Build history of the part. All positions in model axes, mm. Face numbers are marked on the shaded views. A direction names the side the tool comes from. Coordinates: 2 decimals unless noted, no trailing zeros. Loops run counter-clockwise (first coordinate to the right, second up) from the corner with the lowest first, then second, coordinate; pieces in that order, holes last.
Item 1: 3-axis set-ups, long thin cutter, end or side, ignore diameter. For the marked faces 1, 2 and 3: which of +Z, -Z, +X, -X, +Y, -Y reach the whole face in a straight line?
Item 2: Cut at A-A (y = 0.5). List the corners of the cut face in (x, z).
Item 3: Mould opens along X. For the marked faces 4, 5, 6 and 7 say: released by +X, released by -X, zero draft, split by the parting line, or undercut.
Item 4: Flat gauge pins, fed straight in: pin 1 (1.8 mm diameter, centred on x = -14, y = -28.5, fed in from -Z); pin 2 (3 mm diameter, centred on x = 14, y = -28.5, fed in from -Z); pin 3 (3 mm diameter, centred on y = -25, z = 1, fed in from +X); pin 4 (1.8 mm diameter, centred on y = -25.5, z = 2.5, fed in from -X). Where does each tip first touch, or does it go through?
Item 5: Cut at B-B (z = 0.7). List the corners of the cut face in (x, y).
Item 6: Drill centre lines: line 1 along X through (y, z) = (-25, 5.4); line 2 along Y through (x, z) = (-14, 2.6); line 3 along X through (y, z) = (5.5, 1.4). Where is each one in solid material? Low to high.
Item 7: Cut at C-C (x = -14). List the corners of the cut face in (y, z), and give its area (3 significant figures).
Item 8: Cut at D-D (x = -0.5). List the corners of the cut face in (y, z), and give its area (3 significant figures).
from build123d import *

# Parameters (mm, degrees)
F0_R     = 1
F0_W     = 23
F0_H     = 6
F1_DEPTH = 6


# Not quite as in the source:
# - a feature names something its author has since deleted; it is built from what else it names


with BuildPart() as f1:
    # F0 (on Top) → F1 (new body)
    with BuildSketch(Plane.XY):
        with BuildLine():
            Line((-16.5, -21.0738723458), (-16.5, -14.1520673478))
            ThreePointArc((-16.5, -14.1520673478), (-17.620350525, -10.9095454242), (-18, -7.5))
            Line((-18, -7.5), (-18, 9))
            Line((-18, 9), (-10.5, 9))
            Line((-10.5, 9), (-10.5, 13.0000002682))
            Line((-10.5, 13.0000002682), (-22.0000002682, 13.0000002682))
            Line((-22.0000002682, 13.0000002682), (-22.0000002682, -7.5))
            ThreePointArc((-22.0000002682, -7.5), (-20.5727697686, -14.8229094869), (-16.5, -21.0738723458))
        make_face()
        with BuildLine():
            Line((14.3321600082, -23), (11.4999999106, -23))
            Line((11.5, -23), (11.5, -24.7988442176))
            ThreePointArc((11.4999999553, -24.7988442176), (12.9548401383, -23.9604473859), (14.3321600082, -23))
        make_face()
        with BuildLine():
            ThreePointArc((14.3321600082, -23), (12.9548401383, -23.9604473859), (11.4999999553, -24.7988442176))
            Line((11.5, -24.7988442176), (11.5, -29))
            Line((11.4999999106, -29), (11.4999999106, -35))
            Line((11.4999999106, -35), (11.4999999106, -41))
            Line((11.4999999106, -41), (16.4999999106, -41))
            Line((16.4999999106, -41), (16.4999999106, -23))
            Line((16.4999999106, -23), (14.3321600082, -23))
        make_face()
        with Locations((14, -28.5)):
            Circle(F0_R, mode=Mode.SUBTRACT)
        with BuildLine():
            ThreePointArc((18, -7.5), (17.620350525, -10.9095454242), (16.5, -14.1520673478))
            Line((16.5, -14.1520673478), (16.5, -21.0738723458))
            ThreePointArc((16.5, -21.0738723458), (20.5727697686, -14.8229094869), (22.0000002682, -7.5))
            Line((22.0000002682, -7.5), (22.0000002682, 13.0000002682))
            Line((22.0000002682, 13.0000002682), (10.5, 13.0000002682))
            Line((10.5, 13.0000002682), (10.5, 9))
            Line((10.5, 9), (18, 9))
            Line((18, 9), (18, -7.5))
        make_face()
        with BuildLine():
            Line((-11.5, -24.7988441711), (-11.5, -23))
            Line((-11.5000000894, -23), (-14.3321600082, -23))
            ThreePointArc((-14.3321600082, -23), (-12.9548401808, -23.9604473589), (-11.5000000447, -24.7988441711))
        make_face()
        with BuildLine():
            Line((-11.5, -29), (-11.5, -24.7988441711))
            ThreePointArc((-11.5000000447, -24.7988441711), (-12.9548401808, -23.9604473589), (-14.3321600082, -23))
            Line((-14.3321600082, -23), (-16.5000000894, -23))
            Line((-16.5000000894, -23), (-16.5000000894, -41))
            Line((-16.5000000894, -41), (-11.5000000894, -41))
            Line((-11.5000000894, -41), (-11.5000000894, -35))
            Line((-11.5000000894, -35), (-11.5000000894, -29))
        make_face()
        with Locations((-14, -28.5)):
            Circle(F0_R, mode=Mode.SUBTRACT)
        with BuildLine():
            Line((-16.5000000894, -23), (-14.3321600082, -23))
            ThreePointArc((-14.3321600082, -23), (-15.4519347824, -22.0772904153), (-16.5, -21.0738723458))
            Line((-16.5, -21.0738723458), (-16.5, -23))
        make_face()
        with Locations((-8.94e-08, -38)):
            Rectangle(F0_W, F0_H)
        with BuildLine():
            ThreePointArc((16.5, -21.0738723458), (15.4519347824, -22.0772904153), (14.3321600082, -23))
            Line((14.3321600082, -23), (16.4999999106, -23))
            Line((16.5, -23), (16.5, -21.0738723458))
        make_face()
        with BuildLine():
            ThreePointArc((16.5, -14.1520673478), (14.3807555592, -17.4547801253), (11.5, -20.1194294641))
            Line((11.5, -20.1194294641), (11.5, -23))
            Line((11.4999999106, -23), (14.3321600082, -23))
            ThreePointArc((14.3321600082, -23), (15.4519347824, -22.0772904153), (16.5, -21.0738723458))
            Line((16.5, -21.0738723458), (16.5, -14.1520673478))
        make_face()
        with BuildLine():
            Line((-11.5, -23), (-11.5, -20.1194294641))
            ThreePointArc((-11.5, -20.1194294641), (-14.3807555592, -17.4547801253), (-16.5, -14.1520673478))
            Line((-16.5, -14.1520673478), (-16.5, -21.0738723458))
            ThreePointArc((-16.5, -21.0738723458), (-15.4519347824, -22.0772904153), (-14.3321600082, -23))
            Line((-14.3321600082, -23), (-11.5000000894, -23))
        make_face()
    extrude(amount=F1_DEPTH)


solid = f1.part
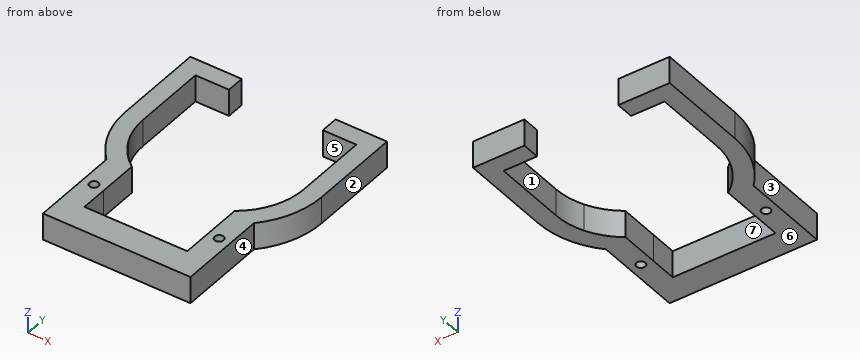
Filled sheet:
1. face 1: +Z, -Z
1. face 2: +Z, -Z, +X, +Y, -Y
1. face 3: +Z, -Z, -X, -Y
2. outline: (-22, 0) - (-18, 0) - (-18, 6) - (-22, 6) - close; (18, 0) - (22, 0) - (22, 6) - (18, 6) - close
3. face 4: released by +X
3. face 5: undercut
3. face 6: zero draft
3. face 7: undercut
4. pin 1: passes through
4. pin 2: stops at z = 0
4. pin 3: stops at x = 16.5
4. pin 4: stops at x = -16.5
5. outline: (-22, -7.5) arc R19.5 ccw to (-16.5, -21.07) - (-16.5, -41) - (16.5, -41) - (16.5, -21.07) arc R19.5 ccw to (22, -7.5) - (22, 13) - (10.5, 13) - (10.5, 9) - (18, 9) - (18, -7.5) arc R15.5 cw to (11.5, -20.12) - (11.5, -35) - (-11.5, -35) - (-11.5, -20.12) arc R15.5 cw to (-18, -7.5) - (-18, 9) - (-10.5, 9) - (-10.5, 13) - (-22, 13) - close; hole circle Ø2 at (-14, -28.5); hole circle Ø2 at (14, -28.5)
6. line 1: x = -16.5 to -11.5, 11.5 to 16.5
6. line 2: y = -41 to -29.5, -27.5 to -17.89, 9 to 13
6. line 3: x = -22 to -18, 18 to 22
7. outline: (-41, 0) - (-29.5, 0) - (-29.5, 6) - (-41, 6) - close; (-27.5, 0) - (-17.89, 0) - (-17.89, 6) - (-27.5, 6) - close; (9, 0) - (13, 0) - (13, 6) - (9, 6) - close
7. area: 151 mm2
8. outline: (-41, 0) - (-35, 0) - (-35, 6) - (-41, 6) - close
8. area: 36.0 mm2
